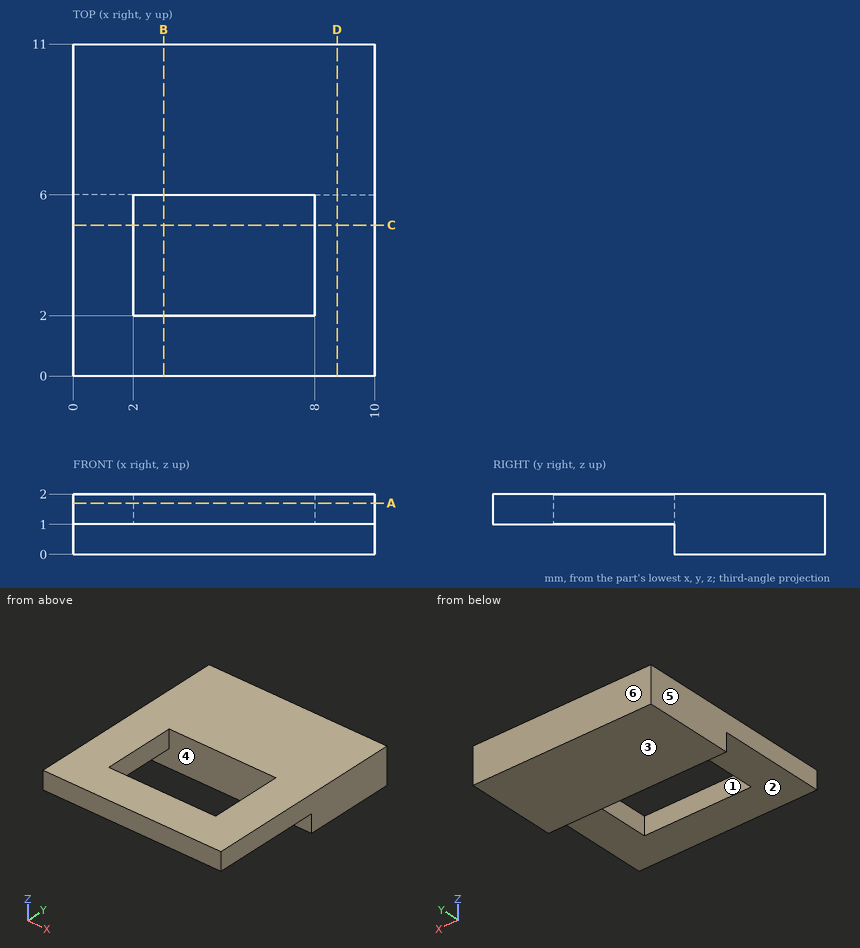
Can you work these out from the drawing? Everything is in mm from the part's minimum corner. A direction names the side the tool comes from. Coordinates: 2 decimals unless noted, no trailing zeros. Loops run counter-clockwise (first coordinate to the right, second up) from the corner with the lowest first, then second, coordinate; pieces in that order, holes last. Notation, with made-up numbers: (-36.75, -25) - (-28.75, -25) arc R4 cw to (-28.75, -20) - close; hole circle Ø9 at (-19.75, 82.5). An arc over 180 degrees is marked (long way). Answer as CSV lines item,"result".
Q1. If we section it at A-A, the plane z = 1.7: Write out the boundary of the cut face in (x, y), and give its area (3 significant figures).
Response:
outline,"(0, 0) - (10, 0) - (10, 11) - (0, 11) - close; hole (2, 2) - (8, 2) - (8, 6) - (2, 6) - close"
area,"86.0 mm2"
Q2. If we section it at C-C, the plane y = 5: Write out the boundary of the cut face in (x, z), and give its area (3 significant figures).
Response:
outline,"(0, 1) - (2, 1) - (2, 2) - (0, 2) - close; (8, 1) - (10, 1) - (10, 2) - (8, 2) - close"
area,"4.00 mm2"
Q3. If I drill on L1, parallel to Y at x = 2.75, z = 1.25; L2, parallel to Y at x = 2.5, z = 0.7; L3, parallel to Z at x = 8, y = 0.75, over which ranges is the centre line in solid material (lowest first)? Write a range as [from, to].
Response:
L1,"[0, 2], [6, 11]"
L2,"[6, 11]"
L3,"[1, 2]"
Q4. If we section it at B-B, the plane x = 3: Write out the boundary of the cut face in (y, z), and give its area (3 significant figures).
Response:
outline,"(0, 1) - (2, 1) - (2, 2) - (0, 2) - close; (6, 0) - (11, 0) - (11, 2) - (6, 2) - close"
area,"12.0 mm2"
Q5. We'd pull the mould along X, two halves only. Please class the marked faces 4, 5 and 6: pulls with the +X half, pulls with the -X half, needs draft (parallel to the pull), parting line crosses it, or undercut.
Response:
face 4,"undercut"
face 5,"pulls with the -X half"
face 6,"needs draft"
Q6. If we section it at D-D, the plane x = 8.75: Write out the boundary of the cut face in (y, z), and give its area (3 significant figures).
Response:
outline,"(0, 1) - (6, 1) - (6, 0) - (11, 0) - (11, 2) - (0, 2) - close"
area,"16.0 mm2"
Q7. For the marked faces 1, 2 and 3, which set-ups out of +Z, -Z, +X, -X, +Y, -Y let a thin tool reach every point of the face, with its end or its side?
Response:
face 1,"+Z, -Z"
face 2,"-Z, +X, -X, -Y"
face 3,"-Z, +X, -X, +Y, -Y"
